Job drawing, mm, ordinate dimensions from the low corner. One solid piece. A direction names the side the tool comes from. Give positions to 0.01 mm unless a question says otherwise; leave off trailing zeros. Order: outer loops, then holes, each group sorted by start corner. A loop starts at its lowest first (then second) coordinate and runs counter-clockwise, first axis right, second up.
1. Mould opens along Z. For the marked faces 3, 4 and 5 say: +Z half, -Z half, draft (parallel to the pull), parting line (faces both ways), or undercut.
2. Probe line 1 (X direction, y = 37.6, z = 43); line 2 (Z direction, x = 70, y = 37.85); line 3 (Z direction, x = 12, y = 31). List the from-to ranges inside material, lowest first.
3. Drop flat-ended pins along their axis: pin 1 Ø13.5 at (x, z) = (39.5, 20.5) entering from -Y; pin 2 Ø4 at (y, z) = (11, 53.5) entering from +X; pin 3 Ø7.5 at (x, z) = (15, 29.5) entering from -Y; pin 4 Ø2 at (x, z) = (70, 12) entering from -Y. Give the stop position or say it passes through.
4. Which spindle directions (+Z, -Z, +X, -X, +Y, -Y) get a long thin tool onto all of the face, cutting with end or side? Do the marked faces 1 and 2. Say none if no direction does.
5. Slice it at C-C on y = 19.5. List the corners of the cut face in (x, z), and give its area (3 significant figures).
6. Slice it at A-A on y = 31.5. List the corners of the cut face in (x, z).
7. Slice it at B-B on x = 12. List the corners of the cut face in (y, z).
8. Slice it at D-D on z = 43. List the corners of the cut face in (x, y), and give its area (4 significant figures).
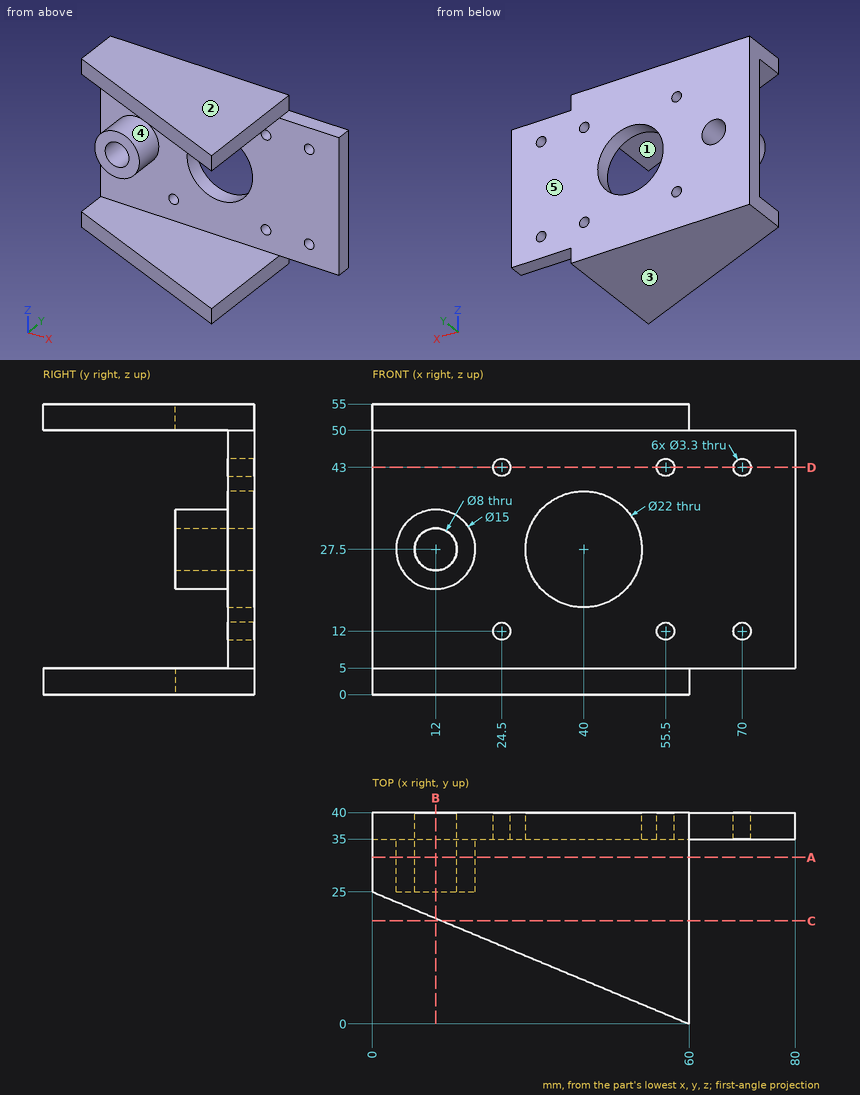
Data:
1. face 3: -Z half
1. face 4: undercut
1. face 5: draft
2. line 1: x = 0 to 22.85, 26.15 to 53.85, 57.15 to 68.35, 71.65 to 80
2. line 2: z = 5 to 10.35, 13.65 to 41.35, 44.65 to 50
2. line 3: z = 0 to 5, 20 to 23.5, 31.5 to 35, 50 to 55
3. pin 1: stops at y = 35
3. pin 2: stops at x = 60
3. pin 3: stops at y = 25
3. pin 4: passes through
4. face 1: +X, -X, -Y
4. face 2: +Z, +X, -X, +Y, -Y
5. outline: (13.2, 0) - (60, 0) - (60, 5) - (13.2, 5) - close; (13.2, 50) - (60, 50) - (60, 55) - (13.2, 55) - close
5. area: 468 mm2
6. outline: (0, 0) - (60, 0) - (60, 5) - (0, 5) - close; (0, 50) - (60, 50) - (60, 55) - (0, 55) - close; circle Ø15 at (12, 27.5); hole circle Ø8 at (12, 27.5)
7. outline: (20, 0) - (40, 0) - (40, 23.5) - (25, 23.5) - (25, 20) - (35, 20) - (35, 5) - (20, 5) - close; (20, 50) - (35, 50) - (35, 35) - (25, 35) - (25, 31.5) - (40, 31.5) - (40, 55) - (20, 55) - close
8. outline: (0, 35) - (22.85, 35) - (22.85, 40) - (0, 40) - close; (26.15, 35) - (53.85, 35) - (53.85, 40) - (26.15, 40) - close; (57.15, 35) - (68.35, 35) - (68.35, 40) - (57.15, 40) - close; (71.65, 35) - (80, 35) - (80, 40) - (71.65, 40) - close
8. area: 350.5 mm2
